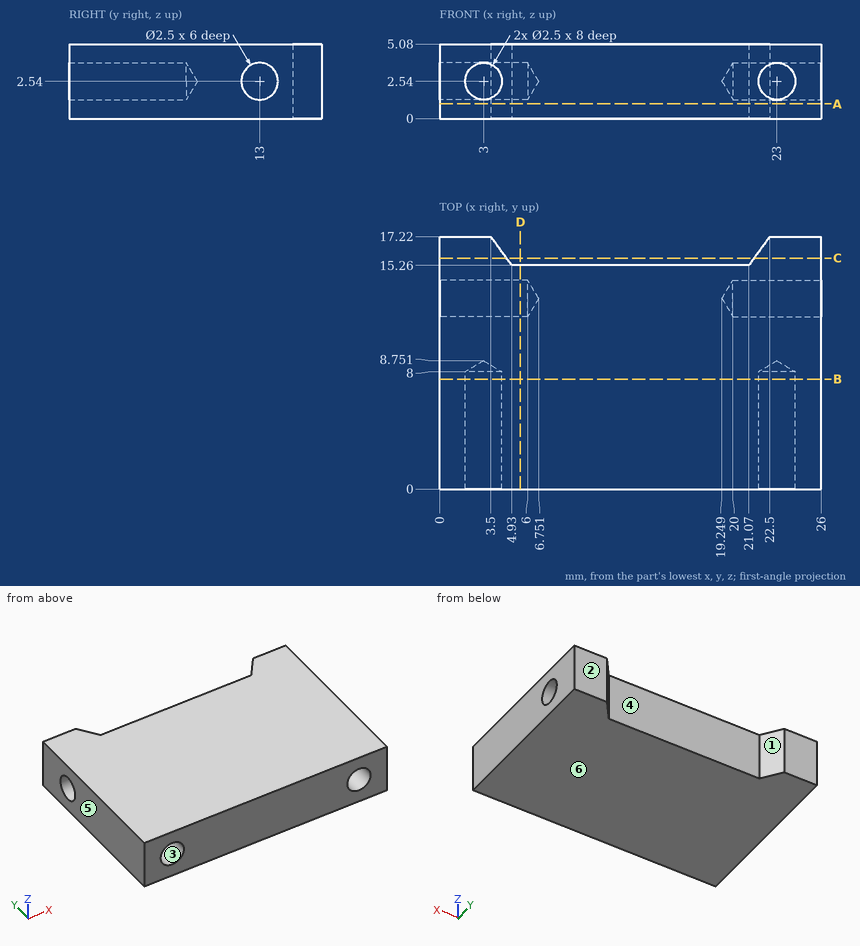
Job drawing, mm, ordinate dimensions from the low corner. One solid piece. A direction names the side the tool comes from. Coordinates: 2 decimals unless noted, no trailing zeros. Order: outer loops, then holes, each group sorted by start corner. A loop starts at its lowest first (then second) coordinate and runs counter-clockwise, first axis right, second up. Notation, with made-up numbers: (65.25, -22.75) -> (105.25, -22.75) arc R8 ccw to (105.25, -7.75) -> close; hole circle Ø2 at (73.5, 24). An arc over 180 degrees is marked (long way). Return JSON: item names as keys, results as strings. Group by question number.
Item 1: Saw through at A-A on z = 1. Write the cut outline in (x, y), then the cut area to 3 significant figures.
Item 2: Flat gauge pins, fed straight in: P1, Ø2, axis at x = 15.5, z = 1.5, coming from the +Y side; P2, Ø2, axis at x = 23, z = 2.54, coming from the -Y side. Where does each tip first touch, or does it go through?
Item 3: Tool access for the marked faces 1, 2 and 3: list every direction of +Z, -Z, +X, -X, +Y, -Y with a clear straight run to the whole face (end or side of a thin tool).
Item 4: Saw through at C-C on y = 15.75. Write the cut outline in (x, z), then the cut area to 3 significant figures.
Item 5: Pull direction X, two halves, no side cores. Call the marked faces 4, 5 and 6: pulls with the +X half, pulls with the -X half, needs draft (parallel to the pull), parting line crosses it, or undercut.
Item 6: Saw through at D-D on x = 5.5. Write the cut outline in (y, z).
Item 7: Wall check: line 1 along X through (y, z) = (2, 2.6); line 2 along Z through (x, y) = (3, 5); line 3 along Y through (x, z) = (7, 0.45). Give the ranges that are in metal, low to high. Write a range as [from, to].
Item 8: Saw through at B-B on y = 7.5. Write the cut outline in (x, z).
Values found:
{
 "1": {"outline": "(0, 0) -> (26, 0) -> (26, 17.22) -> (22.5, 17.22) -> (21.07, 15.26) -> (4.93, 15.26) -> (3.5, 17.22) -> (0, 17.22) -> close", "area": "413 mm2"},
 "2": {"P1": "stops at y = 15.26", "P2": "stops at y = 8.15"},
 "3": {"face 1": "+Z, -Z, +Y", "face 2": "+Z, -Z, +X, -X, +Y", "face 3": "-Y"},
 "4": {"outline": "(0, 0) -> (4.57, 0) -> (4.57, 5.08) -> (0, 5.08) -> close; (21.43, 0) -> (26, 0) -> (26, 5.08) -> (21.43, 5.08) -> close", "area": "46.5 mm2"},
 "5": {"face 4": "undercut", "face 5": "pulls with the -X half", "face 6": "needs draft"},
 "6": {"outline": "(0, 0) -> (15.26, 0) -> (15.26, 5.08) -> (0, 5.08) -> close; hole circle Ø2.5 at (13, 2.54)"},
 "7": {"line 1": "x = [0, 1.75], [4.25, 21.75], [24.25, 26]", "line 2": "z = [0, 1.29], [3.79, 5.08]", "line 3": "y = [0, 15.26]"},
 "8": {"outline": "(0, 0) -> (26, 0) -> (26, 5.08) -> (0, 5.08) -> close; hole circle Ø2.5 at (3, 2.54); hole circle Ø2.5 at (23, 2.54)"}
}
